Source: CAD feature listing. Evaluate the final solid. Frame: model axes, mm. A direction names the side the tool comes from. Give positions to 0.01 mm unless a question says otherwise; leave off trailing zeros. Order: outer loops, then holes, each group sorted by start corner. A loop starts at its lowest first (then second) coordinate and runs counter-clockwise, first axis right, second up.
```python
from build123d import *

# Parameters (mm, degrees)
PAD_DEPTH       = 2.5
CHAMFER_SIZE    = 1
SKETCH001_R     = 1.1
POCKET_DEPTH    = 12
CHAMFER001_SIZE = 0.3


with BuildPart() as part:
    # Sketch → Pad (new body, symmetric)
    with BuildSketch(Plane.XY):
        with BuildLine():
            Line((-29.17, 0), (-29.17, 35))
            ThreePointArc((-24.17, 40), (-27.705534, 38.535534), (-29.17, 35))
            Line((-24.17, 40), (24.17, 40))
            ThreePointArc((29.17, 35), (27.705534, 38.535534), (24.17, 40))
            Line((29.17, 35), (29.17, 0))
            Line((29.17, 0), (24.17, 0))
            Line((24.17, 20), (24.17, 0))
            ThreePointArc((24.17, 20), (21.241068, 27.071068), (14.17, 30))
            Line((-14.17, 30), (14.17, 30))
            ThreePointArc((-14.17, 30), (-21.241068, 27.071068), (-24.17, 20))
            Line((-24.17, 0), (-24.17, 20))
            Line((-29.17, 0), (-24.17, 0))
        make_face()
    extrude(amount=PAD_DEPTH, both=True)

    # Chamfer
    chamfer_edges = [part.edges().sort_by_distance(p)[0] for p in [
        (-26.67, 0, 2.5),
        (-29.17, 17.5, 2.5),
        (-27.705534, 38.535534, 2.5),
        (0, 40, 2.5),
        (27.705534, 38.535534, 2.5),
        (29.17, 17.5, 2.5),
        (26.67, 0, 2.5),
        (24.17, 10, 2.5),
        (21.241068, 27.071068, 2.5),
        (0, 30, 2.5),
        (-21.241068, 27.071068, 2.5),
        (-24.17, 10, 2.5),
        (-26.67, 0, -2.5),
        (-29.17, 17.5, -2.5),
        (-27.705534, 38.535534, -2.5),
        (0, 40, -2.5),
        (27.705534, 38.535534, -2.5),
        (29.17, 17.5, -2.5),
        (26.67, 0, -2.5),
        (24.17, 10, -2.5),
        (21.241068, 27.071068, -2.5),
        (0, 30, -2.5),
        (-21.241068, 27.071068, -2.5),
        (-24.17, 10, -2.5),
        (-29.17, 0, 0),
        (-24.17, 0, 0),
        (24.17, 0, 0),
        (29.17, 0, 0),
    ]]
    chamfer(chamfer_edges, length=CHAMFER_SIZE)

    # Sketch001 → Pocket (cut)
    with BuildSketch(Plane.XZ):
        with Locations((-26.67, 0)):
            Circle(SKETCH001_R)
        with Locations((26.67, 0)):
            Circle(SKETCH001_R)
    extrude(amount=-POCKET_DEPTH, mode=Mode.SUBTRACT)

    # Chamfer001
    chamfer001_edges = [part.edges().sort_by_distance(p)[0] for p in [
        (-27.77, 0, 0),
        (25.57, 0, 0),
    ]]
    chamfer(chamfer001_edges, length=CHAMFER001_SIZE)


solid = part.part
```
1) Reachability of faces 5 (the conical face through (21.275, 27.263, 1.66)), 6 (the conical face through (-27.22, 37.99, -2.23)), 7 (the flat face through (24.17, 11, 0)), 8 (the flat face through (-27, 12, 0)), 9 (the conical face through (21.28, 27.27, -1.67)) from +Z, -Z, +X, -X, +Y, -Y: full face, straight path, thin tool, end or side. Return the list, or none.
Report:
face 5: +Z, -Y
face 6: -Z, -X, +Y
face 7: +Z, -Z, -Y
face 8: -Y
face 9: -Z, -Y
2) Draft query along X for faces 1 (the flat face through (2, 33, -2.5)), 2 (the cylindrical face through (27.74, 38.5, 0.02)), 3 (the cylindrical face through (21.32, 26.99, 0.02)), 4 (the conical face through (-27.22, 37.99, 2.23)). Return one class per face: +X half, -X half, draft (parallel to the pull), parting line (faces both ways), or undercut.
Report:
face 1: draft
face 2: +X half
face 3: undercut
face 4: -X half
3) Section query A-A, the plane y = 13. Return the cut outline in (x, z), and give its area (3 significant figures).
Report:
outline: (-29.17, -1.5) - (-28.17, -2.5) - (-25.17, -2.5) - (-24.17, -1.5) - (-24.17, 1.5) - (-25.17, 2.5) - (-28.17, 2.5) - (-29.17, 1.5) - close; (24.17, -1.5) - (25.17, -2.5) - (28.17, -2.5) - (29.17, -1.5) - (29.17, 1.5) - (28.17, 2.5) - (25.17, 2.5) - (24.17, 1.5) - close
area: 46.0 mm2
4) Pin query (flat end, axial travel): pin 1 (10 mm diameter, centred on x = -6, y = 29.5, fed in from -Z); pin 2 (3 mm diameter, centred on x = 26.67, z = 0, fed in from +Y); pin 3 (0.7 mm diameter, centred on x = 27, z = 0, fed in from -Y); pin 4 (1.5 mm diameter, centred on x = -3, z = 0, fed in from -Y). Return the tip coordinate at first contact, or that it passes through.
Report:
pin 1: stops at z = -2.5
pin 2: stops at y = 39.9
pin 3: stops at y = 12
pin 4: stops at y = 30
5) Section query B-B, the plane x = 0. Return the cut outline in (y, z).
Report:
outline: (30, -1.5) - (31, -2.5) - (39, -2.5) - (40, -1.5) - (40, 1.5) - (39, 2.5) - (31, 2.5) - (30, 1.5) - close
6) Material intervals for L1, parallel to X at y = 2.5, z = 0.05; L2, parallel to Z at x = -26.67, y = 9.5; L3, parallel to X at y = 16.5, z = -0.15, sorted ascending.
Report:
L1: x = -29.17 to -27.77, -25.57 to -24.17, 24.17 to 25.57, 27.77 to 29.17
L2: z = -2.5 to -1.1, 1.1 to 2.5
L3: x = -29.17 to -24.17, 24.17 to 29.17
7) Section query C-C, the plane z = 0. Return the cut outline in (x, y).
Report:
outline: (-29.17, 1) - (-28.17, 0) - (-28.07, 0) - (-27.77, 0.3) - (-27.77, 12) - (-25.57, 12) - (-25.57, 0.3) - (-25.27, 0) - (-25.17, 0) - (-24.17, 1) - (-24.17, 20) arc R10 cw to (-14.17, 30) - (14.17, 30) arc R10 cw to (24.17, 20) - (24.17, 1) - (25.17, 0) - (25.27, 0) - (25.57, 0.3) - (25.57, 12) - (27.77, 12) - (27.77, 0.3) - (28.07, 0) - (28.17, 0) - (29.17, 1) - (29.17, 35) arc R5 ccw to (24.17, 40) - (-24.17, 40) arc R5 ccw to (-29.17, 35) - close
